Can you work these out from the model? Positions are in its coordinate system, mm. Face numbers are marked on the shaded views. A direction names the side the tool comes from. Round coordinates to 2 decimals unless told otherwise and drop trailing zeros. Loops run counter-clockwise (first coordinate to the right, second up) from the corner with the lowest first, then second, coordinate; pieces in that order, holes last. Notation, with made-up numbers: (11, 13.5) -> (39, 13.5) arc R29 ccw to (39, 51.5) -> close; hole circle Ø2 at (2.25, 52). An arc over 180 degrees is marked (long way). Write item = value, one per line.
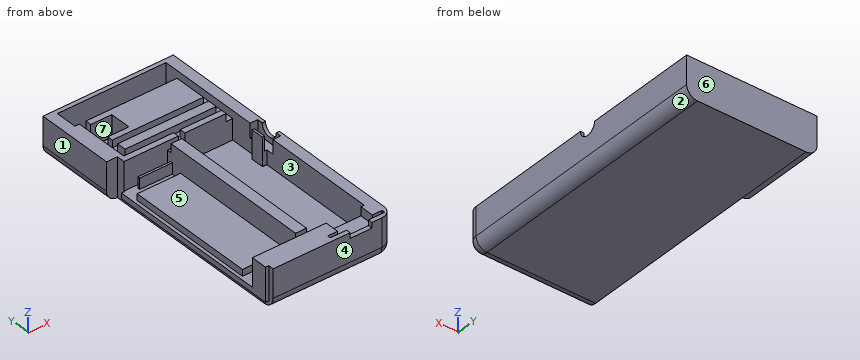
from build123d import *

# Parameters (mm, degrees)
F0_W      = 20
F0_H      = 75
F0_W_2    = 25
F1_DEPTH  = 13
F2_DEPTH  = 5
F3_R      = 4
F4_DEPTH  = 5
F5_W      = 3.5
F5_H      = 13
F6_DEPTH  = 6.5
F7_W      = 88.7834078074
F7_H      = 18
F8_DEPTH  = 5
F10_DEPTH = 5
F11_W     = 1.2834078074
F11_H     = 13
F12_DEPTH = 5
F13_W     = 3
F13_H     = 2.6685215533
F13_H_2   = 1.2419745326
F13_W_2   = 0.7530017495
F13_H_3   = 3
F14_DEPTH = 3.5
F15_W     = 5
F15_H     = 2
F16_DEPTH = 4
F17_W     = 15
F17_H     = 1
F18_DEPTH = 5
F19_R     = 5
F20_W     = 10
F20_H     = 2.5
F21_DEPTH = 10
F22_W     = 16
F22_H     = 4
F23_DEPTH = 8
F24_W     = 25
F24_H     = 1.5
F25_DEPTH = 4
F27_DEPTH = 3.5
F28_W     = 2
F28_H     = 6
F29_DEPTH = 13
F30_W     = 1
F30_H     = 6
F31_DEPTH = 6.5
F32_W     = 1.6611641645
F32_H     = 2.5
F33_DEPTH = 1.5
F35_DEPTH = 3.5
F36_DEPTH = 25
F37_W     = 50
F37_H     = 10
F38_DEPTH = 15
F39_R     = 5
F40_W     = 9.7111338079
F40_H     = 9.7418390214
F41_DEPTH = 10
F42_DEPTH = 3.5
F40_W_2   = 3
F40_H_2   = 15.0616638362
F43_DEPTH = 3.5
F44_W     = 60
F44_H     = 3
F45_DEPTH = 20


with BuildPart() as f1:
    # F0 (on Top) → F1 (new body)
    with BuildSketch(Plane.XY):
        Polygon((-26.3411931316, 47.0243954659), (-46.3411931316, 47.0243954659), (-46.3411931316, -52.9756045341), (13.6588068684, -52.9756045341), (13.6588068684, 47.0243954659), (-6.3411931316, 47.0243954659), align=None)
        with Locations((-31.3411931316, -5.4756045341)):
            Rectangle(F0_W, F0_H, mode=Mode.SUBTRACT)
        with Locations((-3.8411931316, -5.4756045341)):
            Rectangle(F0_W_2, F0_H, mode=Mode.SUBTRACT)
    extrude(amount=F1_DEPTH)

    # F0 (on Top) → F2 (join)
    with BuildSketch(Plane.XY):
        Polygon((-26.3411931316, 47.0243954659), (-46.3411931316, 47.0243954659), (-46.3411931316, -52.9756045341), (13.6588068684, -52.9756045341), (13.6588068684, 47.0243954659), (-6.3411931316, 47.0243954659), align=None)
        with Locations((-31.3411931316, -5.4756045341)):
            Rectangle(F0_W, F0_H, mode=Mode.SUBTRACT)
        with Locations((-3.8411931316, -5.4756045341)):
            Rectangle(F0_W_2, F0_H, mode=Mode.SUBTRACT)
        with Locations((-3.8411931316, -5.4756045341)):
            Rectangle(F0_W_2, F0_H)
        with Locations((-31.3411931316, -5.4756045341)):
            Rectangle(F0_W, F0_H)
    extrude(amount=-F2_DEPTH)

    # F3 (on face) → F4 (cut)
    with BuildSketch(Plane.YZ.offset(13.6588068684)):
        with Locations((15.5341364443, 13)):
            Circle(F3_R)
    extrude(amount=-F4_DEPTH, mode=Mode.SUBTRACT)

    # F5 (on face) → F6 (cut)
    with BuildSketch(Plane.XY.offset(13)):
        with Locations((10.4088068684, 15.5341364443)):
            Rectangle(F5_W, F5_H)
    extrude(amount=-F6_DEPTH, mode=Mode.SUBTRACT)

    # F7 (on face) → F8 (cut)
    with BuildSketch(Plane(origin=(-46.3411931316, 0, 0), x_dir=(0, -1, 0), z_dir=(-1, 0, 0))):
        with Locations((8.5839006305, 4)):
            Rectangle(F7_W, F7_H)
    extrude(amount=-F8_DEPTH, mode=Mode.SUBTRACT)

    # F9 (on face) → F10 (join)
    with BuildSketch(Plane(origin=(-41.3411931316, 0, 0), x_dir=(0, -1, 0), z_dir=(-1, 0, 0))):
        Polygon((-33.3078032732, 13), (-33.3078032732, -2.5), (50.4756045341, -2.5), (50.4756045341, 13), (42.9756045341, 13), (42.9756045341, 0), (-32.0243954659, 0), (-32.0243954659, 13), align=None)
    extrude(amount=F10_DEPTH)

    # F11 (on face) → F12 (cut)
    with BuildSketch(Plane(origin=(-46.3411931316, 0, 0), x_dir=(0, -1, 0), z_dir=(-1, 0, 0))):
        with Locations((-32.6660993695, 6.5)):
            Rectangle(F11_W, F11_H)
    extrude(amount=-F12_DEPTH, mode=Mode.SUBTRACT)

    # F13 (on face) → F14 (cut)
    with BuildSketch(Plane.XY.offset(13)):
        Polygon((5.6588068684, 32.0243954659), (8.6588068684, 32.0243954659), (8.6588068684, 42.0243954659), (5.6588068684, 42.0243954659), (5.6588068684, 37.6929170191), (5.6588068684, 34.6929170191), align=None)
        Polygon((-13.3411931316, 34.6929170191), (5.6588068684, 34.6929170191), (5.6588068684, 37.6929170191), (-36.2876081169, 37.6929170191), (-36.2876081169, 34.6929170191), (-16.3411931316, 34.6929170191), (-16.3411931316, 35.9348915517), (-13.3411931316, 35.9348915517), align=None)
        with Locations((-14.8411931316, 33.3586562425)):
            Rectangle(F13_W, F13_H)
        with Locations((-14.8411931316, 35.3139042854)):
            Rectangle(F13_W, F13_H_2)
        with Locations((-36.6641089916, 36.1929170191)):
            Rectangle(F13_W_2, F13_H_3)
        Polygon((-37.0406098664, 37.6929170191), (-36.2876081169, 37.6929170191), (-36.2876081169, 41.9627316296), (-39.2876081169, 41.9627316296), (-39.2876081169, 34.6929170191), (-37.0406098664, 34.6929170191), align=None)
    extrude(amount=-F14_DEPTH, mode=Mode.SUBTRACT)

    # F15 (on face) → F16 (cut)
    with BuildSketch(Plane.XY.offset(13)):
        with Locations((-18.8411931316, 31.0243954659)):
            Rectangle(F15_W, F15_H)
        with Locations((-18.8411931316, -41.9756045341)):
            Rectangle(F15_W, F15_H)
    extrude(amount=-F16_DEPTH, mode=Mode.SUBTRACT)

    # F17 (on face) → F18 (join)
    with BuildSketch(Plane.XY):
        with Locations((-28.8411931316, 29.7873775363)):
            Rectangle(F17_W, F17_H)
    extrude(amount=F18_DEPTH)

    # F19
    f19_edges = [f1.edges().sort_by_distance(p)[0] for p in [
        (13.658807, -2.975605, -5),
        (-13.841193, -52.975605, -5),
        (13.658807, -52.975605, 4),
        (-46.341193, 41.416099, -5),
    ]]
    fillet(f19_edges, radius=F19_R)

    # F20 (on face) → F21 (cut)
    with BuildSketch(Plane.XZ.offset(52.9756045341)):
        with Locations((-0.8757225672, 11.75)):
            Rectangle(F20_W, F20_H)
    extrude(amount=-F21_DEPTH, mode=Mode.SUBTRACT)

    # F22 (on face) → F23 (cut)
    with BuildSketch(Plane(origin=(0, -42.9756045341, 0), x_dir=(-1, 0, 0), z_dir=(0, 1, 0))):
        with Locations((0.8757225672, 11)):
            Rectangle(F22_W, F22_H)
    extrude(amount=-F23_DEPTH, mode=Mode.SUBTRACT)

    # F24 (on face) → F25 (cut)
    with BuildSketch(Plane.XY.offset(13)):
        with Locations((-0.8757225672, -50.2256045341)):
            Rectangle(F24_W, F24_H)
    extrude(amount=-F25_DEPTH, mode=Mode.SUBTRACT)

    # F26 (on face) → F27 (cut)
    with BuildSketch(Plane(origin=(-46.3411931316, 0, 0), x_dir=(0, -1, 0), z_dir=(-1, 0, 0))):
        Polygon((-33.3078032732, 0), (-33.3078032732, -2.5), (50.4756045341, -2.5), (50.4756045341, 13), (42.9756045341, 13), (42.9756045341, 0), align=None)
    extrude(amount=-F27_DEPTH, mode=Mode.SUBTRACT)

    # F28 (on face) → F29 (join)
    with BuildSketch(Plane.XY):
        with Locations((7.6588068684, 15.5341364443)):
            Rectangle(F28_W, F28_H)
    extrude(amount=F29_DEPTH)

    # F30 (on face) → F31 (cut)
    with BuildSketch(Plane.XY.offset(13)):
        with Locations((8.1588068684, 15.5341364443)):
            Rectangle(F30_W, F30_H)
    extrude(amount=-F31_DEPTH, mode=Mode.SUBTRACT)

    # F32 (on face) → F33 (cut)
    with BuildSketch(Plane(origin=(-42.8411931316, 0, 0), x_dir=(0, -1, 0), z_dir=(-1, 0, 0))):
        with Locations((-32.4772211909, -1.25)):
            Rectangle(F32_W, F32_H)
    extrude(amount=-F33_DEPTH, mode=Mode.SUBTRACT)

    # F34 (on face) → F35 (cut)
    with BuildSketch(Plane.XY.offset(13)):
        Polygon((-39.2876081169, 44.9627316296), (-39.2876081169, 41.9627316296), (-36.2876081169, 41.9627316296), (5.6588068684, 41.9627316296), (5.6588068684, 42.0243954659), (8.6588068684, 42.0243954659), (8.6588068684, 44.9627316296), align=None)
    extrude(amount=-F35_DEPTH, mode=Mode.SUBTRACT)

    # F36 (add): a face of the model
    f36_faces = [f1.faces().sort_by_distance(p)[0] for p in [
        (-16.3411931316, 47.0243954659, 4.07910728),
    ]]
    extrude(f36_faces, amount=F36_DEPTH)

    # F37 (on face) → F38 (cut)
    with BuildSketch(Plane.XY.offset(13)):
        with Locations((-16.3411931316, 65.0243954659)):
            Rectangle(F37_W, F37_H)
    extrude(amount=-F38_DEPTH, mode=Mode.SUBTRACT)

    # F39
    f39_edges = [f1.edges().sort_by_distance(p)[0] for p in [
        (8.658807, 65.024395, -2),
        (-41.341193, 65.024395, -2),
    ]]
    fillet(f39_edges, radius=F39_R)

    # F40 (on face) → F41 (cut)
    with BuildSketch(Plane.XY.offset(13)):
        with Locations((-31.4320412129, 52.4028521031)):
            Rectangle(F40_W, F40_H)
    extrude(amount=-F41_DEPTH, mode=Mode.SUBTRACT)

    # F40 (on face) → F42 (cut)
    with BuildSketch(Plane.XY.offset(13)):
        Polygon((-39.2876081169, 60.0243954659), (-39.2876081169, 44.9627316296), (-36.2876081169, 44.9627316296), (-36.2876081169, 47.5319325924), (-36.2876081169, 57.2737716138), (-36.2876081169, 60.0243954659), align=None)
    extrude(amount=-F42_DEPTH, mode=Mode.SUBTRACT)

    # F40 (on face) → F43 (cut)
    with BuildSketch(Plane.XY.offset(13)):
        with Locations((7.1588068684, 52.4935635477)):
            Rectangle(F40_W_2, F40_H_2)
    extrude(amount=-F43_DEPTH, mode=Mode.SUBTRACT)

    # F44 (on face) → F45 (join)
    with BuildSketch(Plane(origin=(-21.3411931316, 0, 0), x_dir=(0, -1, 0), z_dir=(-1, 0, 0))):
        with Locations((5.4616580904, 1.5)):
            Rectangle(F44_W, F44_H)
    extrude(amount=F45_DEPTH)


solid = f1.part
1. Suppose I cut it at C-C, the plane z = 1.25. Count the separate pieces of the cut face and the enclosed holes in it, and give its area (3 significant figures).
Entries:
separate_pieces = 1
enclosed_holes = 2
area = 4,420 mm²
2. For the marked faces 5, 6 and 7, which set-ups out of +Z, -Z, +X, -X, +Y, -Y let a thin tool reach every point of the face, with its end or its side?
Entries:
face_5 = +Z, -X
face_6 = +Z, -Z, +X, -X, +Y
face_7 = +Z
3. I'm going to push flat-ended pins straight in: pin 1 (1.2 mm diameter, centred on y = -50.5, z = 10, fed in from +X); pin 2 (0.6 mm diameter, centred on x = -17.5, y = -41.5, fed in from +Z); pin 3 (2 mm diameter, centred on y = -52, z = 12, fed in from -X). Where does each tip first touch, or does it pass through?
Entries:
pin_1 = 13.27
pin_2 = 9
pin_3 = -41.34
4. I need wall thicknesses on line 1 (Y direction, x = -1, z = 8); line 2 (Y direction, x = -22.5, z = 11); line 3 (Y direction, x = -32.5, z = 1.5). Which ranges of each line are inside material? Lowest first, please. Write a range as [from, to].
Entries:
line_1 = [-52.98, -42.98], [32.02, 60.02], [70.02, 72.02]
line_2 = [-52.98, -42.98], [32.02, 34.69], [37.69, 41.96], [44.96, 60.02], [70.02, 72.02]
line_3 = [-52.98, -42.98], [-35.46, 24.54], [29.29, 30.29], [32.02, 60.02], [70.02, 72.02]
5. Suppose I cut it at D-D, the plane x = -18. List the corners of the cut face in (y, z) for me, and give its area (3 significant figures).
Entries:
outline = (-52.98, 0) arc R5 ccw to (-47.98, -5) -> (72.02, -5) -> (72.02, 13) -> (70.02, 13) -> (70.02, -2) -> (60.02, -2) -> (60.02, 13) -> (44.96, 13) -> (44.96, 9.5) -> (41.96, 9.5) -> (41.96, 13) -> (37.69, 13) -> (37.69, 9.5) -> (34.69, 9.5) -> (34.69, 13) -> (32.02, 13) -> (32.02, 9) -> (30.02, 9) -> (30.02, 13) -> (-40.98, 13) -> (-40.98, 9) -> (-42.98, 9) -> (-42.98, 13) -> (-52.98, 13) -> close
area = 2,060 mm²
6. Suppose I cut it at A-A, the plane y = 40.5. List the corners of the cut face in (x, z) for me, and give its area (3 significant figures).
Entries:
outline = (-46.34, 0) arc R5 ccw to (-41.34, -5) -> (8.66, -5) arc R5 ccw to (13.66, 0) -> (13.66, 13) -> (8.66, 13) -> (8.66, 9.5) -> (5.66, 9.5) -> (5.66, 13) -> (-36.29, 13) -> (-36.29, 9.5) -> (-39.29, 9.5) -> (-39.29, 13) -> (-46.34, 13) -> close
area = 1,050 mm²
7. We'd pull the mould along X, two halves only. Please class the marked faces 1, 2, 3 and 4: released by +X, released by -X, zero draft, split by the parting line, or undercut.
Entries:
face_1 = released by -X
face_2 = released by +X
face_3 = undercut
face_4 = zero draft
